The model under review builds one solid part; all positions refer to its coordinate system, in mm. Face numbers are marked on the shaded views. Round coordinates to 2 decimals unless told otherwise and drop trailing zeros. Order: outer loops, then holes, each group sorted by start corner. A loop starts at its lowest first (then second) coordinate and runs counter-clockwise, first axis right, second up.
1) Consider section A-A (y = 16.75). Give the number of separate pieces and of enclosed holes in the cut face, then the cut area to 3 significant figures.
2) Clearance check with flat-ended pins moving along their axes: P1, Ø13.5, axis at x = -99, z = 85.5, coming from the +Y side; P2, Ø3.5, axis at y = 9.525, z = 38.1, coming from the -X side; P3, Ø2.5, axis at y = 9.525, z = 38.1, coming from the -X side. State where each tip first meets the part, or that it passes through.
3) Mouldability with a two-part tool opening along X and no side actions: class the marked faces 1, 2, 3 and 4 as pulls with the +X half, pulls with the -X half, needs draft (parallel to the pull), parting line crosses it, or undercut.
4) Consider section B-B (x = -106). Give the boundary of the cut face in (y, z), then the cut area to 3 significant figures.
5) To check wall thickness, follow L1, parallel to X at y = 5.25, z = 57; L2, parallel to Z at x = -39, y = 5.25; L3, parallel to X at y = 14.75, z = 83.5. State the ranges of each line that lie inside material, in increasing order.
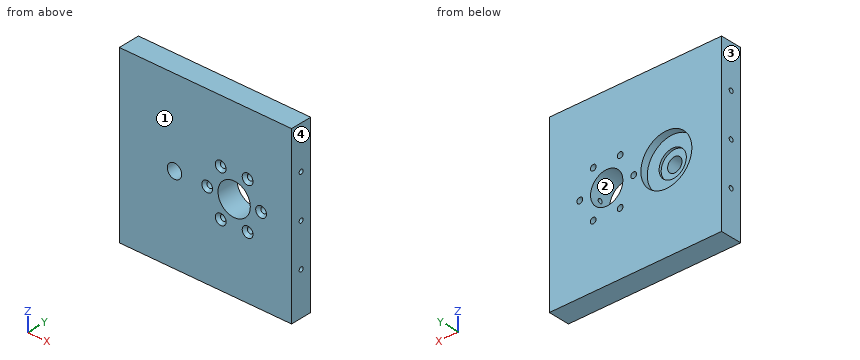
Autodesk Inventor part; units mm, degrees
ref_plane "Work Plane1" through (-76.2, 0, 0) normal (-1, 0, 0) x (0, 0, 1)
ref_plane "YZ Plane" through (0, 0, 0) normal (1, 0, 0) x (0, 1, 0)
ref_plane "XZ Plane" through (0, 0, 0) normal (0, 1, 0) x (-1, 0, 0)
sketch "Sketch1" plane through (0, 0, 0) normal (0, 1, 0) x (-1, 0, 0)
  line L0 (0, 0) -> (152.4, 0)
  line L1 (152.4, 0) -> (152.4, 152.4)
  line L2 (152.4, 152.4) -> (0, 152.4)
  line L3 (0, 152.4) -> (0, 0)
  dimension "d0" = 152.4
  dimension "d1" = 152.4
extrude "Extrusion1" add sketch "Sketch1" along normal blind 12.7
hole "Hole1" at (-103.5558, 12.7, 76.2) direction (0, -1, 0) diameter 12.7 end through all
hole "Hole2" at (-50.8, 12.7, 76.2) direction (0, -1, 0) diameter 28.575 end through all
hole "Hole3" at (38.1, 0, 58.6994) direction (0, 1, 0) diameter 4.5 end through all countersink diameter 9.525 countersink angle 82
pattern_circular "Circular Pattern1" count 4 over 360 about axis through (-103.5558, -203.2, 76.2) along (0, 1, 0) of "Hole3"
sketch "Sketch4" plane through (0, 12.7, 0) normal (0, 1, 0) x (1, 0, 0)
  circle A0 centre (-103.5558, -76.2) radius 6.35
  circle A1 centre (-103.5558, -76.2) radius 12.0332
  dimension "d41" = 24.0665
sketch "Sketch5" plane through (0, 12.7, 0) normal (0, 1, 0) x (1, 0, 0)
  circle A0 centre (-50.8, -76.2) radius 14.2875
  circle A1 centre (-103.5558, -76.2) radius 6.35
  line L0 (0, 0) -> (-152.4, 0)
  line L1 (-152.4, 0) -> (-152.4, -152.4)
  line L2 (-152.4, -152.4) -> (0, -152.4)
  line L3 (0, -152.4) -> (0, 0)
  circle A2 centre (-103.5558, -76.2) radius 22.5425
  dimension "d42" = 45.085
extrude "Extrusion4" add sketch "Sketch5" along normal blind 6.35 contours L3 L2 L1 L0
extrude "Extrusion5" cut sketch "Sketch4" against normal blind 2.032
hole "Hole4" at (-26.9748, 0, 76.2) direction (0, 1, 0) diameter 5.08 end through all countersink diameter 9.525 countersink angle 82
pattern_circular "Circular Pattern2" count 6 over 360 about axis through (-50.8, 19.05, 76.2) along (0, -1, 0) of "Hole4"
hole "Hole5" at (0, 9.525, 114.3) direction (-1, 0, 0) diameter 3.9624 depth 38.1 tip angle 118
pattern_linear "Rectangular Pattern1" count 3 spacing 38.1 along (0, 0, -1) of "Hole5"
ref_plane "Work Plane1" through (-76.2, 0, 0) normal (-1, 0, 0) x (0, 0, 1)
mirror "Mirror1" about plane through (-76.2, 0, 0) normal (-1, 0, 0) of "Hole5", "Rectangular Pattern1"
properties part number "Traveler"
Answer below:
1. separate pieces: 1
1. enclosed holes: 8
1. area: 20,900 mm2
2. P1: stops at y = 12.7
2. P2: stops at x = -114.16
2. P3: stops at x = -113.86
3. face 1: needs draft
3. face 2: undercut
3. face 3: pulls with the -X half
3. face 4: pulls with the +X half
4. outline: (0, 0) - (19.05, 0) - (19.05, 53.79) - (12.7, 53.79) - (12.7, 64.42) - (10.67, 64.42) - (10.67, 70.34) - (0, 70.34) - close; (0, 82.06) - (10.67, 82.06) - (10.67, 87.98) - (12.7, 87.98) - (12.7, 98.61) - (19.05, 98.61) - (19.05, 152.4) - (0, 152.4) - close
4. area: 2,450 mm2
5. L1: x = -152.4 to -64.81, -60.62 to -40.98, -36.79 to 0
5. L2: z = 0 to 53.03, 58.1 to 68.14, 84.26 to 94.3, 99.37 to 152.4
5. L3: x = -152.4 to -124.88, -82.23 to -63.08, -38.52 to 0
